Geometry check sheet. Reference: the model listing, model coordinates, mm. A direction names the side the tool comes from. Coordinates: 2 decimals unless noted, no trailing zeros. Loops run counter-clockwise (first coordinate to the right, second up) from the corner with the lowest first, then second, coordinate; pieces in that order, holes last.
from build123d import *

# Parameters (mm, degrees)
F1_DEPTH = 5
F2_DEPTH = 5
F3_COUNT = 16
F5_D     = 6


with BuildPart() as f1:
    # F0 (on Top) → F1 (new body)
    with BuildSketch(Plane.XY):
        with BuildLine():
            ThreePointArc((-2.5837804825, 11.9744134895), (-7.6945171742, -9.5318888713), (12.25, 0))
            ThreePointArc((12.25, 0), (8.7317956514, 8.59175446), (0.1980416814, 12.2483990583))
            ThreePointArc((0.1980416814, 12.2483990583), (-1.200709969, 12.1910129017), (-2.5837804825, 11.9744134895))
        make_face()
    extrude(amount=F1_DEPTH)

    # F0 (on Top) → F2 (join)
    with BuildSketch(Plane.XY):
        with BuildLine():
            ThreePointArc((-2.5837804825, 11.9744134895), (-1.200709969, 12.1910129017), (0.1980416814, 12.2483990583))
            ThreePointArc((0.1980416814, 12.2483990583), (0.208626449, 13.1365918946), (0, 14))
            ThreePointArc((0, 14), (-0.5553297077, 14.953396215), (-1.3770560583, 15.6896850387))
            Line((-1.3770560583, 15.6896850387), (-1.7103093943, 15.6568624499))
            ThreePointArc((-1.7103093943, 15.6568624499), (-2.3726036798, 14.7744103512), (-2.7312645082, 13.7309939256))
            ThreePointArc((-2.7312645082, 13.7309939256), (-2.7674396932, 12.8434749638), (-2.5837804825, 11.9744134895))
        make_face()
    extrude(amount=F2_DEPTH)

    # F3: F1 ×16 about axis
    f3_axis = Axis((0, 0, 5), (0, 0, -1))


with BuildPart() as f1_1:
    add(f1.part)
    for i in range(1, F3_COUNT):
        add(f1.part.rotate(f3_axis, i * 360 / F3_COUNT))

    # F5 (through all)
    with Locations(Plane(origin=(0, 0, 0), x_dir=(1, 0, 0), z_dir=(0, 0, -1))):
        with Locations((0, 0)):
            Hole(F5_D / 2)


solid = f1_1.part
1) Section check A-A on y = 14.5. Record the cut outline in (x, z), and give its area (3 significant figures).
Data:
outline: (-2.5, 0) - (-0.24, 0) - (-0.24, 5) - (-2.5, 5) - close; (3.39, 0) - (5.03, 0) - (5.03, 5) - (3.39, 5) - close
area: 19.5 mm2
2) Access from +Z, -Z, +X, -X, +Y, -Y to the whole of each face (thin tool, end or side, straight path). Record for faces 5 (the cylindrical face through (7.76, -9.48, 2.46)), 6 (the cylindrical face through (-8.78, -12.13, 2.46)), 7 (the cylindrical face through (14.941, 0.546, 2.465)).
Data:
face 5: +Z, -Z
face 6: +Z, -Z, -Y
face 7: +Z, -Z, +X
3) Material ranges on probe 1 along Y at (x, z) = (-12, 3.2); probe 2 along X at (y, z) = (-13.5, 2.45); probe 3 along X at (y, z) = (14.5, 2.6), recorded low to high.
Data:
probe 1: y = -7.84 to -4.72, -2.59 to 5.2, 8.43 to 10.13
probe 2: x = -5.32 to -2.6, -0.15 to 2.76, 6.06 to 7.69
probe 3: x = -2.5 to -0.24, 3.39 to 5.03
4) Depth check by flat-ended pin: pin 1 (3 mm diameter, centred on x = -4, z = 3.5, fed in from -Y); pin 2 (2 mm diameter, centred on y = -3, z = 0.5, fed in from -X); pin 3 (2 mm diameter, centred on y = 0.5, z = 2, fed in from -X). Enter the tip coordinate at first touch or a pass-through.
Data:
pin 1: stops at y = -15.12
pin 2: stops at x = -15.34
pin 3: stops at x = -14.88
5) Section check B-B on x = 6. Record the cut outline in (y, z).
Data:
outline: (-13.46, 0) - (10.68, 0) - (10.68, 5) - (-13.46, 5) - close
6) Mould release check, pull along X, two halves, no side actions. Record for faces 1 (the cylindrical face through (7.844, -12.757, 2.465)), 2 (the cylindrical face through (5.787, 10.797, 2.465)), 3 (the cylindrical face through (-13.12, 0.21, 2.46)), 4 (the cylindrical face through (-13.595, -6.222, 2.465)): +X half, -X half, draft (parallel to the pull), parting line (faces both ways), or undercut.
Data:
face 1: +X half
face 2: undercut
face 3: undercut
face 4: -X half
